For this review, use the dimensioned drawing (mm, ordinates from the lowest corner) and the shaded views. A direction names the side the tool comes from. Round coordinates to 2 decimals unless told otherwise and drop trailing zeros. Order: outer loops, then holes, each group sorted by start corner. A loop starts at its lowest first (then second) coordinate and runs counter-clockwise, first axis right, second up. Notation, with made-up numbers: M 57.25,-3 L 67.25,-3 A24 cw 67.25,27 Z; hole C 6.5,-17.5 d5. An arc over 180 degrees is marked long. Put each result on its own line as item: value.
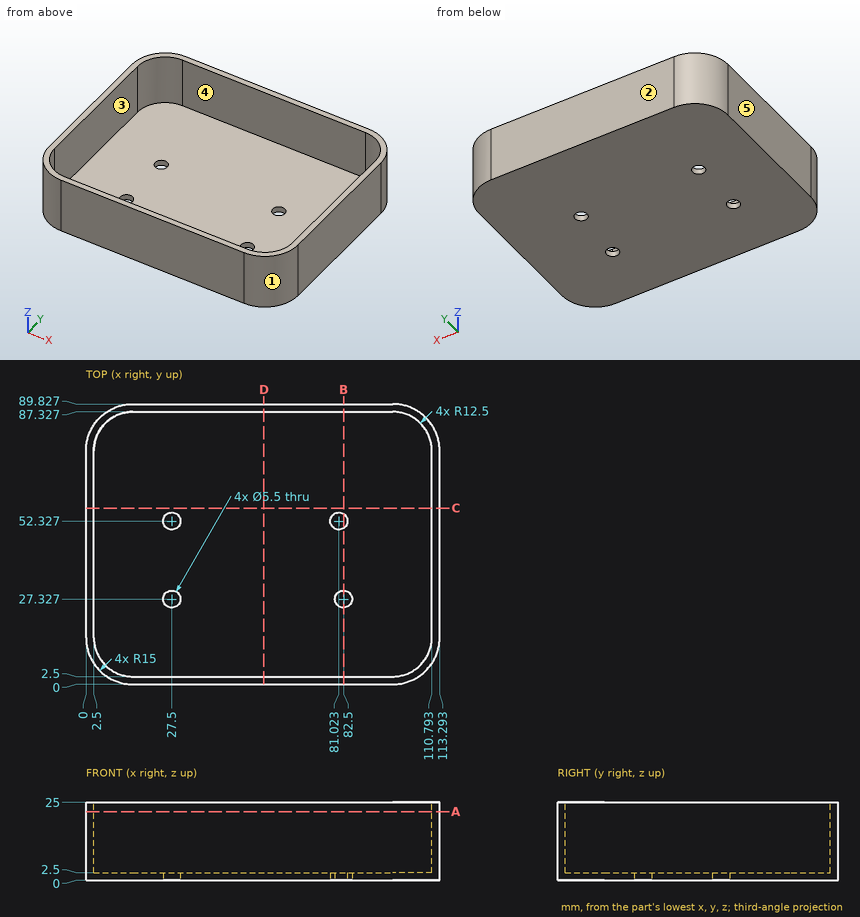
(1) For the marked faces 4 and 5, list the 3-axis set-ups (+Z, -Z, +X, -X, +Y, -Y) from which the entire face can be reached by the end or side of a thin tool; tool diameter is ignored.
A:
face 4: +Z
face 5: +Z, -Z, -X, +Y, -Y
(2) To check wall thickness, follow L1, parallel to Y at x = 27.5, z = 1.95; L2, parallel to Y at x = 45.5, z = 3; L3, parallel to X at y = 50.5, z = 1.5 (1 decimal). State the ranges of each line that lie inside material, in increasing order.
A:
L1: y = 0 to 24.58, 30.08 to 49.58, 55.08 to 89.83
L2: y = 0 to 2.5, 87.33 to 89.83
L3: x = 0 to 25.4, 29.6 to 79, 83.1 to 113.3
(3) Insertion check: pin 1 Ø5 at (y, z) = (73, 18) entering from -X; pin 2 Ø1 at (x, y) = (94.5, 69) entering from +Z; pin 3 Ø3.5 at (x, y) = (27.5, 27.33) entering from +Z. Each pin has a flat end and moves straight along its axis. Give the tip position at first contact, or say it passes through.
A:
pin 1: stops at x = 0
pin 2: stops at z = 2.5
pin 3: passes through
(4) Add section B-B on x = 82.5. Give the boundary of the cut face in (y, z).
A:
outline: M 0,0 L 24.58,0 L 24.58,2.5 L 2.5,2.5 L 2.5,25 L 0,25 Z; M 30.08,0 L 50.01,0 L 50.01,2.5 L 30.08,2.5 Z; M 54.65,0 L 89.83,0 L 89.83,25 L 87.33,25 L 87.33,2.5 L 54.65,2.5 Z
(5) Draft analysis for pull direction Y (two halves, no side actions). For the marked faces 1, 2 and 3, state which applies: released by +Y, released by -Y, zero draft, split by the parting line, or undercut.
A:
face 1: released by -Y
face 2: released by +Y
face 3: undercut
(6) Add section C-C on y = 56.5. Give the boundary of the cut face in (x, z).
A:
outline: M 0,0 L 113.29,0 L 113.29,25 L 110.79,25 L 110.79,2.5 L 2.5,2.5 L 2.5,25 L 0,25 Z
(7) Add section A-A on z = 22. Give the boundary of the cut face in (x, y).
A:
outline: M 0,15 A15 ccw 15,0 L 98.29,0 A15 ccw 113.29,15 L 113.29,74.83 A15 ccw 98.29,89.83 L 15,89.83 A15 ccw 0,74.83 Z; hole M 2.5,15 A12.5 ccw 15,2.5 L 98.29,2.5 A12.5 ccw 110.79,15 L 110.79,74.83 A12.5 ccw 98.29,87.33 L 15,87.33 A12.5 ccw 2.5,74.83 Z
(8) Add section D-D on x = 57. Give the boundary of the cut face in (y, z), then the cut area to 3 significant figures.
A:
outline: M 0,0 L 89.83,0 L 89.83,25 L 87.33,25 L 87.33,2.5 L 2.5,2.5 L 2.5,25 L 0,25 Z
area: 337 mm2
